Can you work these out from the model? Positions are in its coordinate system, mm. A direction names the side the tool comes from. Round coordinates to 2 decimals unless told otherwise and drop trailing zeros. Order: outer loops, then holes, each group sorted by start corner. A loop starts at its lowest first (then second) coordinate and runs counter-clockwise, first axis right, second up. Notation, with made-up numbers: (32, 13) - (60, 13) arc R18 ccw to (60, 22) - close; hole circle Ø8 at (49.5, 26.5). An arc over 180 degrees is marked (long way). Write item = value, one per line.
from build123d import *

# Parameters (mm, degrees)
F1_DEPTH = 65
F0_W     = 65
F0_H     = 8.9540635944
F2_DEPTH = 60
F3_W     = 65
F3_H     = 8.9540635944
F4_DEPTH = 100
F6_DEPTH = 25


with BuildPart() as f1:
    # F0 (on Right) → F1 (new body)
    with BuildSketch(Plane.YZ):
        Polygon((-30, -32.3655755222), (-50, -32.3655755222), (-50, -52.3655755222), (-25, -52.3655755222), (-25, -43.4115119278), (40, -43.4115119278), (40, -52.3655755222), (50, -52.3655755222), (50, -32.3655755222), (30, -32.3655755222), align=None)
    extrude(amount=F1_DEPTH)

    # F0 (on Right) → F2 (join)
    with BuildSketch(Plane.YZ):
        Polygon((-30, -32.3655755222), (-50, -32.3655755222), (-50, -52.3655755222), (-25, -52.3655755222), (-25, -43.4115119278), (40, -43.4115119278), (40, -52.3655755222), (50, -52.3655755222), (50, -32.3655755222), (30, -32.3655755222), align=None)
        with BuildLine():
            Line((-30, -2.3655755222), (-30, -32.3655755222))
            Line((-30, -32.3655755222), (30, -32.3655755222))
            Line((30, -32.3655755222), (30, -2.3655755222))
            Line((30, -2.3655755222), (15, -2.3655755222))
            ThreePointArc((15, -2.3655755222), (0, -17.3655755222), (-15, -2.3655755222))
            Line((-15, -2.3655755222), (-30, -2.3655755222))
        make_face()
        with Locations((7.5, -47.888543725)):
            Rectangle(F0_W, F0_H)
        with BuildLine():
            ThreePointArc((15, -2.3655755222), (0, 12.6344244778), (-15, -2.3655755222))
            Line((-15, -2.3655755222), (-10, -2.3655755222))
            ThreePointArc((-10, -2.3655755222), (0, 7.6344244778), (10, -2.3655755222))
            Line((10, -2.3655755222), (15, -2.3655755222))
        make_face()
        with BuildLine():
            Line((-10, -2.3655755222), (-15, -2.3655755222))
            ThreePointArc((-15, -2.3655755222), (0, -17.3655755222), (15, -2.3655755222))
            Line((15, -2.3655755222), (10, -2.3655755222))
            ThreePointArc((10, -2.3655755222), (0, -12.3655755222), (-10, -2.3655755222))
        make_face()
    extrude(amount=F2_DEPTH)

    # F3 (on face) → F4 (cut)
    with BuildSketch(Plane.YZ.offset(60)):
        with Locations((7.5, -47.888543725)):
            Rectangle(F3_W, F3_H)
    extrude(amount=-F4_DEPTH, mode=Mode.SUBTRACT)

    # F5 (on face) → F6 (cut)
    with BuildSketch(Plane.XY.offset(-32.3655755222)):
        Polygon((65, -35), (55, -50), (65, -50), align=None)
    extrude(amount=-F6_DEPTH, mode=Mode.SUBTRACT)


solid = f1.part
(1) If I drill on line 1 (Z direction, x = 18, y = 0); line 2 (Y direction, x = 41.5, z = -22); line 3 (Z direction, x = 43, y = 27.5), over which ranges is the centre line in solid material (lowest first)? Write a range as from..to.
Computed:
line_1 = -43.41..-12.37, 7.63..12.63
line_2 = -30..30
line_3 = -43.41..-2.37
(2) Will these pins go through, and if not, where does the flat tip stop? P1, Ø7.5, axis at x = 38, y = -20.5, coming from the +Z side; P2, Ø1.5, axis at y = -9, z = -18, coming from the -X side; P3, Ø19.5, axis at x = 16.5, y = -13, coming from the +Z side; P4, Ø6, axis at y = 17, z = -25, coming from the +X side.
Computed:
P1 = -2.37
P2 = 0
P3 = 12.28
P4 = 60
(3) On a 3-axis mill with a long thin cutter (end or side, diameter ignored), from which of +Z, -Z, +X, -X, +Y, -Y can I reach the whole of each face in a straight line? I mean faces 1 (the face through (30, -22, -2.366)), 2 (the face through (29.58, 0.33, 12.63)), 3 (the face through (30, 23, -2.366)), 4 (the face through (33, 40, -48)), 5 (the face through (29.58, 2.168, -12.128)). Say none if no direction works.
Computed:
face_1 = +Z, +X, -X, -Y
face_2 = +Z, +X, -X
face_3 = +Z, +X, -X, +Y
face_4 = -Z, +X, -X
face_5 = +X, -X
(4) If we section it at A-A (y = 0): Write out the boundary of the cut face in (x, z).
Computed:
outline = (0, -43.41) - (65, -43.41) - (65, -32.37) - (60, -32.37) - (60, -12.37) - (0, -12.37) - close; (0, 7.63) - (60, 7.63) - (60, 12.63) - (0, 12.63) - close
(5) Thinking about a two-plate mould opening in Y: for faces 6 (the face through (60.07, -42.395, -42.226)), 7 (the face through (33, -25, -48)), 8 (the face through (60, 0, -15)), which applies, +Y half, -Y half, draft (parallel to the pull), parting line (faces both ways), or undercut?
Computed:
face_6 = -Y half
face_7 = undercut
face_8 = draft
(6) If we section it at D-D (y = 28): Write out the boundary of the cut face in (x, z).
Computed:
outline = (0, -43.41) - (65, -43.41) - (65, -32.37) - (60, -32.37) - (60, -2.37) - (0, -2.37) - close
(7) If we section it at B-B (x = 40.5): Write out the boundary of the cut face in (y, z), plus the area to 3 significant figures.
Computed:
outline = (-50, -52.37) - (-25, -52.37) - (-25, -43.41) - (40, -43.41) - (40, -52.37) - (50, -52.37) - (50, -32.37) - (30, -32.37) - (30, -2.37) - (15, -2.37) arc R15 ccw to (-15, -2.37) - (-30, -2.37) - (-30, -32.37) - (-50, -32.37) - close; hole circle Ø20 at (0, -2.37)
area = 3,260 mm^2
(8) If we section it at C-C (z = 1): Write out the boundary of the cut face in (x, y), plus the area to 3 significant figures.
Computed:
outline = (0, -14.62) - (60, -14.62) - (60, -9.42) - (0, -9.42) - close; (0, 9.42) - (60, 9.42) - (60, 14.62) - (0, 14.62) - close
area = 624 mm^2
